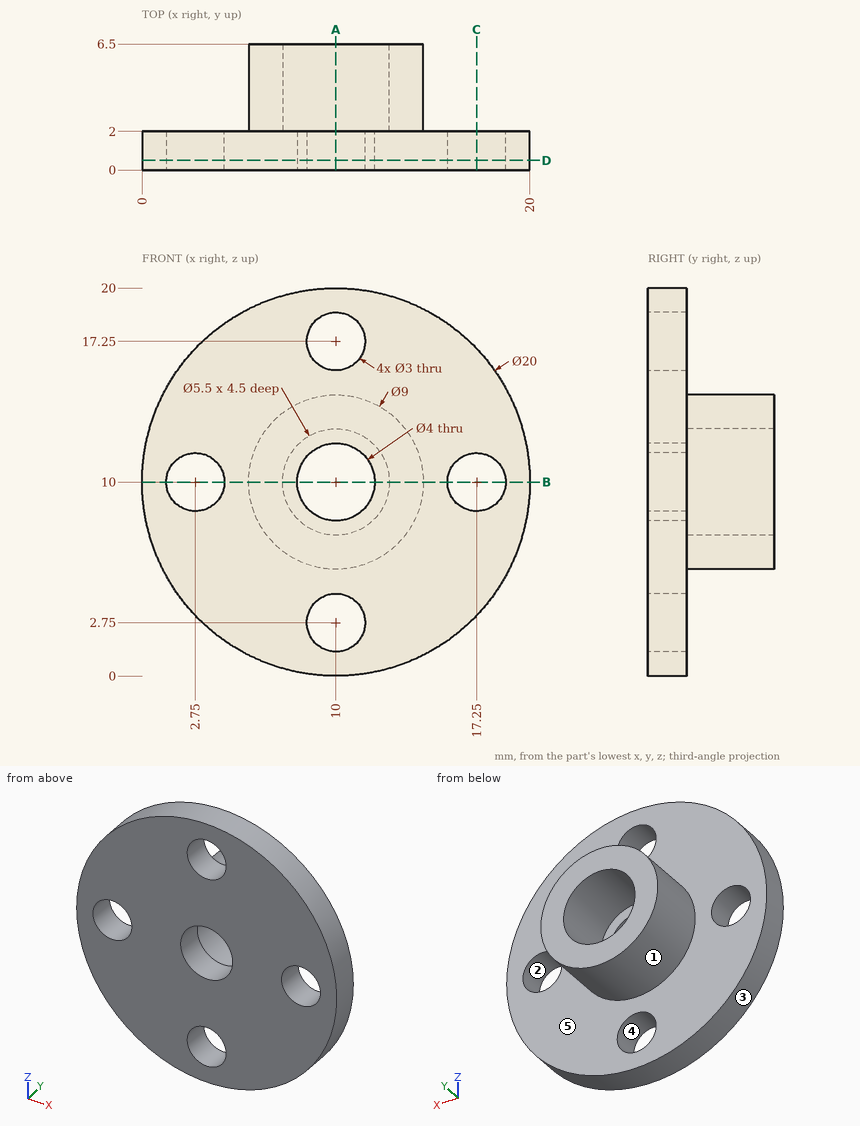
The drawing under review shows one solid part. Ordinate dimensions are in mm from its lowest x, y, z. A direction names the side the tool comes from. Round coordinates to 2 decimals unless told otherwise and drop trailing zeros. Write each loop counter-clockwise with the first axis right and the second up, starting at its lowest first coordinate (ties: lowest second). Pieces come first, ordered by that corner, then holes. Notation, with made-up numbers: (26.25, -1) - (56.25, -1) arc R21 cw to (56.25, 35) - close; hole circle Ø4 at (30.5, 88). An arc over 180 degrees is marked (long way). One line per question, with ' | ' between items.
Item 1: The part is to be moulded in two halves that separate along Z. For the marked faces 3, 4 and 5, say which applies: pulls with the +Z half, pulls with the -Z half, needs draft (parallel to the pull), parting line crosses it, or undercut.
Resolved:
face 3: parting line crosses it | face 4: undercut | face 5: needs draft
Item 2: For the marked faces 1 and 2, list the 3-axis set-ups (+Z, -Z, +X, -X, +Y, -Y) from which the entire face can be reached by the end or side of a thin tool; tool diameter is ignored.
Resolved:
face 1: +Y | face 2: +Y, -Y
Item 3: For P1, Ø3.5, axis at x = 10, z = 17.25, coming from the +Y side; P2, Ø1, axis at y = 1.5, z = 13.5, coming from the -X side; P3, Ø3, axis at y = 4, z = 4.5, coming from the -X side, all flat-tipped, find the tip position at first contact; note any pin that passes through.
Resolved:
P1: stops at y = 2 | P2: stops at x = 0.46 | P3: stops at x = 7.94
Item 4: Add section B-B, the plane z = 10. Give the boundary of the cut face in (x, y), then the cut area to 4 significant figures.
Resolved:
outline: (0, 0) - (1.25, 0) - (1.25, 2) - (0, 2) - close; (4.25, 0) - (8, 0) - (8, 2) - (7.25, 2) - (7.25, 6.5) - (5.5, 6.5) - (5.5, 2) - (4.25, 2) - close; (12, 0) - (15.75, 0) - (15.75, 2) - (14.5, 2) - (14.5, 6.5) - (12.75, 6.5) - (12.75, 2) - (12, 2) - close; (18.75, 0) - (20, 0) - (20, 2) - (18.75, 2) - close | area: 35.75 mm2
Item 5: Add section A-A, the plane x = 10. Give the boundary of the cut face in (y, z).
Resolved:
outline: (0, 0) - (2, 0) - (2, 1.25) - (0, 1.25) - close; (0, 4.25) - (2, 4.25) - (2, 5.5) - (6.5, 5.5) - (6.5, 7.25) - (2, 7.25) - (2, 8) - (0, 8) - close; (0, 12) - (2, 12) - (2, 12.75) - (6.5, 12.75) - (6.5, 14.5) - (2, 14.5) - (2, 15.75) - (0, 15.75) - close; (0, 18.75) - (2, 18.75) - (2, 20) - (0, 20) - close
Item 6: Add section C-C, the plane x = 17.25. Give the boundary of the cut face in (y, z).
Resolved:
outline: (0, 3.11) - (2, 3.11) - (2, 8.5) - (0, 8.5) - close; (0, 11.5) - (2, 11.5) - (2, 16.89) - (0, 16.89) - close
Item 7: To check wall thickness, follow probe 1 along X at (y, z) = (1.2, 10); probe 2 along X at (y, z) = (1.75, 9.5). State the ranges of each line that lie inside material, in increasing order.
Resolved:
probe 1: x = 0 to 1.25, 4.25 to 8, 12 to 15.75, 18.75 to 20 | probe 2: x = 0.01 to 1.34, 4.16 to 8.06, 11.94 to 15.84, 18.66 to 19.99
Item 8: Add section D-D, the plane y = 0.5. Give the boundary of the cut face in (x, z), then the cut area to 3 significant figures.
Resolved:
outline: circle Ø20 at (10, 10); hole circle Ø3 at (2.75, 10); hole circle Ø4 at (10, 10); hole circle Ø3 at (10, 2.75); hole circle Ø3 at (10, 17.25); hole circle Ø3 at (17.25, 10) | area: 273 mm2
